CAD build for the part. Positions are in the model's coordinates, mm. Face numbers are marked on the shaded views. A direction names the side the tool comes from. Coordinates: 2 decimals unless noted, no trailing zeros. Order: outer loops, then holes, each group sorted by start corner. A loop starts at its lowest first (then second) coordinate and runs counter-clockwise, first axis right, second up. Notation, with made-up numbers: (-20.75, 84) - (-8.75, 84) arc R18 cw to (-8.75, 98) - close; hole circle Ø10 at (-3.5, 40). An arc over 180 degrees is marked (long way). Return JSON: item names as keys, results as strings.
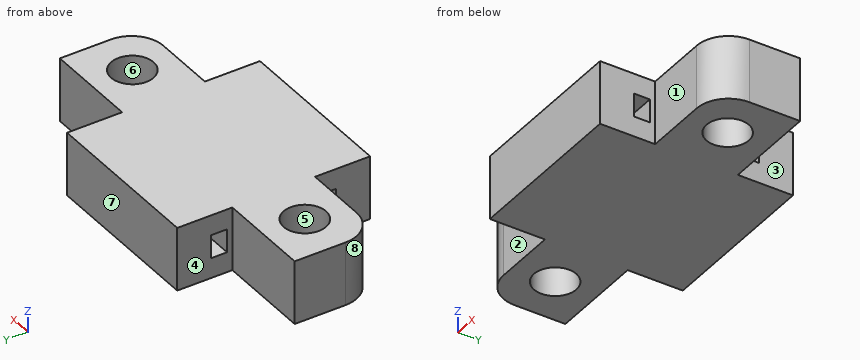
Autodesk Inventor part; units mm, degrees
ref_plane "YZ Plane" through (0, 0, 0) normal (1, 0, 0) x (0, 1, 0)
ref_plane "XZ Plane" through (0, 0, 0) normal (0, 1, 0) x (-1, 0, 0)
ref_plane "XY Plane" through (0, 0, 0) normal (0, 0, 1) x (1, 0, 0)
sketch "Esquisse1" plane through (0, 0, 0) normal (0, 0, 1) x (1, 0, 0)
  line L0 (0, 0) -> (0, 7.8)
  line L1 (0, 7.8) -> (8.97, 7.8)
  line L2 (8.97, 7.8) -> (8.97, 13)
  line L3 (8.97, 13) -> (24.83, 13)
  line L4 (24.83, 13) -> (24.83, 7.8)
  line L5 (24.83, 7.8) -> (33.8, 7.8)
  line L6 (33.8, 7.8) -> (33.8, 0)
  line L7 (33.8, 0) -> (24.83, 0)
  line L8 (24.83, 0) -> (24.83, -5.2)
  line L9 (24.83, -5.2) -> (8.97, -5.2)
  line L10 (8.97, -5.2) -> (8.97, 0)
  line L11 (0, 0) -> (8.97, 0)
  dimension "d0" = 7.8
  dimension "d1" = 7.8
  dimension "d2" = 15.86
  dimension "d3" = 33.8
  dimension "d4" = 18.2
  dimension "d5" = 5.2
  dimension "d6" = 8.97
extrude "Extrusion1" add sketch "Esquisse1" along normal blind 6
sketch "Esquisse2" plane through (0, 0, 6) normal (0, 0, 1) x (1, 0, 0)
  line L0 (0, 7.8) -> (0, 0) construction
  line L1 (0, 0) -> (8.97, 0) construction
  line L2 (0, 7.8) -> (8.97, 0) construction
  line L3 (8.97, 13) -> (8.97, 7.8) construction
  line L4 (8.97, 7.8) -> (0, 0) construction
  line L5 (24.83, 7.8) -> (33.8, 0) construction
  line L6 (33.8, 0) -> (33.8, 7.8) construction
  line L7 (24.83, -5.2) -> (24.83, 0) construction
  line L8 (33.8, 7.8) -> (24.83, 0) construction
  circle A0 centre (4.485, 3.9) radius 2
  circle A1 centre (29.315, 3.9) radius 2
  dimension "d9" = 4
  dimension "d10" = 4
extrude "Extrusion2" cut sketch "Esquisse2" against normal blind 7
fillet "Congé1" radius 3 1 edges at (0, 0, 3)
fillet "Congé2" radius 3 1 edges at (33.8, 0, 3)
sketch "Esquisse3" plane through (24.83, 7.8, 0) normal (1, 0, 0) x (0, 0, -1)
  line L0 (-4.1, 2) -> (-1.9, 2)
  line L1 (-1.9, 2) -> (-1.9, 0.5)
  line L2 (-1.9, 0.5) -> (-4.1, 0.5)
  line L3 (-4.1, 0.5) -> (-4.1, 2)
  line L4 (-4.1, -8.3) -> (-1.9, -8.3)
  line L5 (-1.9, -8.3) -> (-1.9, -9.8)
  line L6 (-1.9, -9.8) -> (-4.1, -9.8)
  line L7 (-4.1, -9.8) -> (-4.1, -8.3)
  line L8 (0, -7.8) -> (-6, -7.8)
  line L9 (0, -7.8) -> (0, -13)
  line L10 (0, 0) -> (-6, 0)
  dimension "d15" = 2.2
  dimension "d16" = 1.5
  dimension "d17" = 0.5
  dimension "d18" = 1.9
  dimension "d19" = 0.5
  dimension "d20" = 1.5
extrude "Extrusion3" cut sketch "Esquisse3" against normal blind 15.86
properties part number "Finger juncture" material "Plastique ABS"
Item 1: Wall check: L1, parallel to Z at x = 17, y = -1.25; L2, parallel to X at y = 9, z = 5.45; L3, parallel to Y at x = 31, z = 2.5. Give the ranges that are in metal, low to high. Write a range as [from, to].
Findings below:
{"L1": "z = [0, 1.9], [4.1, 6]", "L2": "x = [8.97, 24.83]", "L3": "y = [0.01, 2.82], [4.98, 7.8]"}
Item 2: Band-saw the part on C-C, the plane x = 28. List the corners of the cut face in (y, z), then the cut area to 3 significant figures.
Findings below:
{"outline": "(0, 0) - (2.39, 0) - (2.39, 6) - (0, 6) - close; (5.41, 0) - (7.8, 0) - (7.8, 6) - (5.41, 6) - close", "area": "28.7 mm²"}
Item 3: Band-saw the part on B-B, the plane y = 3.9. List the corners of the cut face in (x, z) (3 decimals), then the cut area to 3 significant figures.
Findings below:
{"outline": "(0, 0) - (2.485, 0) - (2.485, 6) - (0, 6) - close; (6.485, 0) - (27.315, 0) - (27.315, 6) - (6.485, 6) - close; (31.315, 0) - (33.8, 0) - (33.8, 6) - (31.315, 6) - close", "area": "155 mm²"}
Item 4: Band-saw the part on A-A, the plane z = 2.9. List the corners of the cut face in (x, y) (3 decimals).
Findings below:
{"outline": "(0, 3) arc R3 ccw to (3, 0) - (8.97, 0) - (8.97, -0.5) - (24.83, -0.5) - (24.83, 0) - (30.8, 0) arc R3 ccw to (33.8, 3) - (33.8, 7.8) - (24.83, 7.8) - (24.83, 8.3) - (8.97, 8.3) - (8.97, 7.8) - (0, 7.8) - close; (8.97, -5.2) - (24.83, -5.2) - (24.83, -2) - (8.97, -2) - close; (8.97, 9.8) - (24.83, 9.8) - (24.83, 13) - (8.97, 13) - close; hole circle Ø4 at (4.485, 3.9); hole circle Ø4 at (29.315, 3.9)"}
Item 5: Band-saw the part on D-D, the plane z = 4.7. List the corners of the cut face in (x, y) (3 decimals).
Findings below:
{"outline": "(0, 3) arc R3 ccw to (3, 0) - (8.97, 0) - (8.97, -5.2) - (24.83, -5.2) - (24.83, 0) - (30.8, 0) arc R3 ccw to (33.8, 3) - (33.8, 7.8) - (24.83, 7.8) - (24.83, 13) - (8.97, 13) - (8.97, 7.8) - (0, 7.8) - close; hole circle Ø4 at (4.485, 3.9); hole circle Ø4 at (29.315, 3.9)"}
Item 6: Mould opens along X. For the marked faces 5, 6, 7 and 8 say: released by +X, released by -X, zero draft, split by the parting line, or undercut.
Findings below:
{"face 5": "undercut", "face 6": "undercut", "face 7": "zero draft", "face 8": "released by -X"}
Item 7: Drop flat-ended pins along their axis: P1, Ø2, axis at x = 14.5, y = 2.5, coming from the -Z side; P2, Ø2.5, axis at y = 11, z = 3.5, coming from the +X side; P3, Ø2.5, axis at x = 29.315, y = 3.9, coming from the -Z side; P4, Ø1.8, axis at x = 28, z = 3.5, coming from the -Y side. Give the stop position or say it passes through.
Findings below:
{"P1": "stops at z = 0", "P2": "stops at x = 24.83", "P3": "passes through", "P4": "stops at y = 0"}
Item 8: Which spindle directions (+Z, -Z, +X, -X, +Y, -Y) get a long thin tool onto all of the face, cutting with end or side? Do the marked faces 1, 2, 3 and 4. Say none if no direction does.
Findings below:
{"face 1": "+Z, -Z, +X, -Y", "face 2": "+Z, -Z, -X, -Y", "face 3": "+Z, -Z, +X, +Y", "face 4": "+Z, -Z, -X, +Y"}
